from build123d import *

# Parameters (mm, degrees)
SKETCH_1_W          = 300
SKETCH_1_H          = 70
SKETCH_1_R          = 7
SKETCH_1_R_2        = 3
SKETCH_1_W_2        = 100
SKETCH_1_H_2        = 30
SKETCH_1_W_3        = 11
SKETCH_1_H_3        = 11
EXTRUDE_1_DEPTH     = 2
FILLET_1_R          = 1.5
FILLET_2_R          = 3
SKETCH_2_R          = 1
CUT_EXTRUDE_1_DEPTH = 155.04220201


with BuildPart() as part:
    # Эскиз1 → Бобышка-Вытянуть1 (new body)
    with BuildSketch(Plane.XY):
        Rectangle(SKETCH_1_W, SKETCH_1_H)
        with Locations((135, 20)):
            Circle(SKETCH_1_R, mode=Mode.SUBTRACT)
        with Locations((135, 0)):
            Circle(SKETCH_1_R, mode=Mode.SUBTRACT)
        with Locations((135, -20)):
            Circle(SKETCH_1_R, mode=Mode.SUBTRACT)
        with Locations((110, 15)):
            Circle(SKETCH_1_R_2, mode=Mode.SUBTRACT)
        with Locations((95, 15)):
            Circle(SKETCH_1_R_2, mode=Mode.SUBTRACT)
        with Locations((80, 15)):
            Circle(SKETCH_1_R_2, mode=Mode.SUBTRACT)
        with Locations((65, 15)):
            Circle(SKETCH_1_R_2, mode=Mode.SUBTRACT)
        with Locations((50, 15)):
            Circle(SKETCH_1_R_2, mode=Mode.SUBTRACT)
        with Locations((30, 15)):
            Circle(SKETCH_1_R_2, mode=Mode.SUBTRACT)
        with Locations((15, 15)):
            Circle(SKETCH_1_R_2, mode=Mode.SUBTRACT)
        with Locations((0, 15)):
            Circle(SKETCH_1_R_2, mode=Mode.SUBTRACT)
        with Locations((-70, 10)):
            Rectangle(SKETCH_1_W_2, SKETCH_1_H_2, mode=Mode.SUBTRACT)
        with Locations((65, 0)):
            Rectangle(SKETCH_1_W_3, SKETCH_1_H_3, mode=Mode.SUBTRACT)
        with Locations((80, 0)):
            Rectangle(SKETCH_1_W_3, SKETCH_1_H_3, mode=Mode.SUBTRACT)
        with Locations((95, 0)):
            Rectangle(SKETCH_1_W_3, SKETCH_1_H_3, mode=Mode.SUBTRACT)
        with Locations((110, 0)):
            Rectangle(SKETCH_1_W_3, SKETCH_1_H_3, mode=Mode.SUBTRACT)
        with Locations((50, 0)):
            Rectangle(SKETCH_1_W_3, SKETCH_1_H_3, mode=Mode.SUBTRACT)
        with Locations((15, 0)):
            Rectangle(SKETCH_1_W_3, SKETCH_1_H_3, mode=Mode.SUBTRACT)
        with Locations((30, 0)):
            Rectangle(SKETCH_1_W_3, SKETCH_1_H_3, mode=Mode.SUBTRACT)
        Rectangle(SKETCH_1_W_3, SKETCH_1_H_3, mode=Mode.SUBTRACT)
        with BuildLine():
            Line((-140, -5), (-140, -15))
            ThreePointArc((-140, -15), (-136, -19), (-132, -15))
            Line((-132, -15), (-132, -5))
            ThreePointArc((-132, -5), (-136, -1), (-140, -5))
        make_face(mode=Mode.SUBTRACT)
    extrude(amount=-EXTRUDE_1_DEPTH)

    # Скругление1
    fillet_1_edges = [part.edges().sort_by_distance(p)[0] for p in [
        (20.5, -5.5, -1),
        (9.5, -5.5, -1),
        (9.5, 5.5, -1),
        (20.5, 5.5, -1),
        (24.5, -5.5, -1),
        (24.5, 5.5, -1),
        (35.5, 5.5, -1),
        (35.5, -5.5, -1),
        (5.5, -5.5, -1),
        (-5.5, -5.5, -1),
        (-5.5, 5.5, -1),
        (5.5, 5.5, -1),
        (59.5, 5.5, -1),
        (70.5, 5.5, -1),
        (70.5, -5.5, -1),
        (59.5, -5.5, -1),
        (74.5, -5.5, -1),
        (74.5, 5.5, -1),
        (85.5, 5.5, -1),
        (85.5, -5.5, -1),
        (89.5, 5.5, -1),
        (100.5, 5.5, -1),
        (100.5, -5.5, -1),
        (89.5, -5.5, -1),
        (104.5, 5.5, -1),
        (115.5, 5.5, -1),
        (115.5, -5.5, -1),
        (104.5, -5.5, -1),
        (44.5, -5.5, -1),
        (44.5, 5.5, -1),
        (55.5, 5.5, -1),
        (55.5, -5.5, -1),
    ]]
    fillet(fillet_1_edges, radius=FILLET_1_R)

    # Скругление2
    fillet_2_edges = [part.edges().sort_by_distance(p)[0] for p in [
        (-120, 25, -1),
        (-20, 25, -1),
        (-20, -5, -1),
        (-120, -5, -1),
    ]]
    fillet(fillet_2_edges, radius=FILLET_2_R)

    # Эскиз2 → Вырез-Вытянуть1 (cut, through all)
    with BuildSketch(Plane.XY):
        with Locations((135, 10)):
            Circle(SKETCH_2_R)
    extrude(amount=-CUT_EXTRUDE_1_DEPTH, mode=Mode.SUBTRACT)


solid = part.part
Input: part model. Units: mm. Frame: model coordinates. Give positions to 0.01 mm unless a question says otherwise; leave off trailing zeros. Order: outer loops, then holes, each group sorted by start corner. A loop starts at its lowest first (then second) coordinate and runs counter-clockwise, first axis right, second up. Notation, with made-up numbers: (51, -20) - (80, -20) arc R25 ccw to (80, 7) - close; hole circle Ø2 at (34.5, 14). An arc over 180 degrees is marked (long way). Answer as a JSON object with one key per item and string values. Group by question number.
Q1. Cut plane A-A, the plane x = 15. Output: boundary loops of the cut face in (y, z), then the cut area to 3 significant figures.
Q2. Cut plane B-B, the plane x = -42. Output: boundary loops of the cut face in (y, z), then the cut area to 3 significant figures.
Q3. Mould query, pull axis X, two halves, no side actions, for faces 1 (the face through (129.84, 4.73, -0.99)), 2 (the face through (-2, -7, 0)). Classes: pulls with the +X half, pulls with the -X half, needs draft (parallel to the pull), parting line crosses it, or undercut.
Q4. Cut plane C-C, the plane z = -0.5. Count the separate pieces of the cut face and the enclosed holes in it, then the cut area to 3 significant figures.
Q5. First-contact query: pin 1 Ø3.5 at (x, y) = (95, 15) entering from +Z. Flat tip, straight axial feed; report the tip coordinate or a pass-through.
Q6. Line query: probe 1 along Y at (x, z) = (80, -1.55); probe 2 along Y at (x, z) = (54, -1.9); probe 3 along X at (y, z) = (-8.5, -0.5). Output: solid intervals per line, ascending.
Results:
{
 "1": {"outline": "(-35, -2) - (-5.5, -2) - (-5.5, 0) - (-35, 0) - close; (5.5, -2) - (12, -2) - (12, 0) - (5.5, 0) - close; (18, -2) - (35, -2) - (35, 0) - (18, 0) - close", "area": "106 mm^2"},
 "2": {"outline": "(-35, -2) - (-5, -2) - (-5, 0) - (-35, 0) - close; (25, -2) - (35, -2) - (35, 0) - (25, 0) - close", "area": "80.0 mm^2"},
 "3": {"face 1": "undercut", "face 2": "needs draft"},
 "4": {"separate pieces": "1", "enclosed holes": "22", "area": "16,200 mm^2"},
 "5": {"pin 1": "through"},
 "6": {"probe 1": "-35 to -5.5, 5.5 to 12, 18 to 35", "probe 2": "-35 to -5.5, 5.5 to 35", "probe 3": "-150 to -140, -132 to 150"}
}
